from build123d import *

# Parameters (mm, degrees)
F0_R          = 5
F0_R_2        = 4.65
F1_DEPTH      = 0.5
F0_R_3        = 1
F0_R_4        = 0.5
F0_R_5        = 0.15
F2_DEPTH      = 1.7
F2_DEPTH_BACK = 1.2
F3_DEPTH      = 3.4
F3_DEPTH_BACK = 2.9
F5_DEPTH      = 0.3
F6_R          = 0.2414213562
F7_SIZE       = 0.05
F8_SIZE       = 0.15
F9_R          = 0.15
F10_DEPTH     = 1


with BuildPart() as f1:
    # F0 (on Top) → F1 (new body)
    with BuildSketch(Plane.XY):
        Circle(F0_R)
        Circle(F0_R_2, mode=Mode.SUBTRACT)
    extrude(amount=F1_DEPTH)



with BuildPart() as f1b:
    # F0 (on Top) → F1, piece 2 (new body)
    with BuildSketch(Plane.XY):
        Circle(F0_R_3)
        Circle(F0_R_4, mode=Mode.SUBTRACT)
    extrude(amount=F1_DEPTH)

    # F0 (on Top) → F2 (join, two sides)
    with BuildSketch(Plane.XY) as f2_sk:
        Circle(F0_R_4)
        Circle(F0_R_5, mode=Mode.SUBTRACT)
    extrude(amount=F2_DEPTH)
    extrude(f2_sk.sketch, amount=-F2_DEPTH_BACK)

    # F0 (on Top) → F3 (join, two sides)
    with BuildSketch(Plane.XY) as f3_sk:
        Circle(F0_R_5)
    extrude(amount=F3_DEPTH)
    extrude(f3_sk.sketch, amount=-F3_DEPTH_BACK)


with BuildPart() as f1_1:
    add(f1.part)

    add(f1b.part)  # F5 merges F1b
    # F4 (on face) → F5 (join)
    with BuildSketch(Plane.XY):
        with BuildLine():
            Line((-0.3600120544, -0.9329476516), (-0.3600120544, -4.6360426358))
            ThreePointArc((-0.3600120544, -4.6360426358), (0, -4.65), (0.3600120544, -4.6360426358))
            Line((0.3600120544, -4.6360426358), (0.3600120544, -0.9329476516))
            ThreePointArc((0.3600120544, -0.9329476516), (0, -1), (-0.3600120544, -0.9329476516))
        make_face()
        with BuildLine():
            ThreePointArc((0.3600120544, 4.6360426358), (0, 4.65), (-0.3600120544, 4.6360426358))
            Line((-0.3600120544, 4.6360426358), (-0.3600120544, 0.9329476516))
            ThreePointArc((-0.3600120544, 0.9329476516), (0, 1), (0.3600120544, 0.9329476516))
            Line((0.3600120544, 0.9329476516), (0.3600120544, 4.6360426358))
        make_face()
    extrude(amount=F5_DEPTH)

    # F6
    f6_edges = [f1_1.edges().sort_by_distance(p)[0] for p in [
        (-0.5, 0, 0.5),
        (-0.5, 0, 0),
        (-0.15, 0, -1.2),
        (-0.15, 0, 1.7),
    ]]
    fillet(f6_edges, radius=F6_R)

    # F7
    f7_edges = [f1_1.edges().sort_by_distance(p)[0] for p in [
        (-5, 0, 0.5),
        (-4.65, 0, 0.5),
        (-4.65, 0, 0),
        (-5, 0, 0),
    ]]
    chamfer(f7_edges, length=F7_SIZE)

    # F8
    f8_edges = [f1_1.edges().sort_by_distance(p)[0] for p in [
        (-0.15, 0, 3.4),
        (-0.15, 0, -2.9),
    ]]
    chamfer(f8_edges, length=F8_SIZE)

    # F9 (on face) → F10 (join)
    with BuildSketch(Plane.XY):
        with Locations((0, -1.5)):
            Circle(F9_R)
    extrude(amount=-F10_DEPTH)


solid = f1_1.part
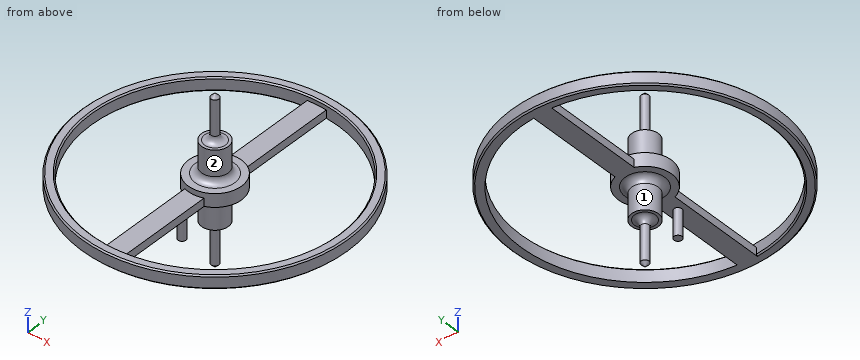
CAD build for the part. Positions are in the model's coordinates, mm. Face numbers are marked on the shaded views. A direction names the side the tool comes from. Give positions to 0.01 mm unless a question says otherwise; leave off trailing zeros. Write each loop counter-clockwise with the first axis right and the second up, starting at its lowest first coordinate (ties: lowest second). Pieces come first, ordered by that corner, then holes. Notation, with made-up numbers: (4, -1.75) -> (31, -1.75) arc R21 cw to (31, 34.25) -> close; hole circle Ø10 at (-0.75, 78.5). An arc over 180 degrees is marked (long way). Return JSON: item names as keys, results as strings.
Item 1: Band-saw the part on B-B (z = 2.5). List the corners of the cut face in (x, y).
Answer below:
{"outline": "circle Ø0.3 at (0, 0)"}
Item 2: Drop flat-ended pins along their axis: pin 1 (3 mm diameter, centred on x = 0, z = 1.5, fed in from -Y); pin 2 (1.5 mm diameter, centred on x = -2, z = 0, fed in from +Y); pin 3 (3 mm diameter, centred on x = -1, y = -3.5, fed in from -Z); pin 4 (5 mm diameter, centred on x = -2, y = 3.5, fed in from +Z). Give the stop position or say it passes through.
Answer below:
{"pin 1": "stops at y = -5", "pin 2": "stops at y = 4.84", "pin 3": "stops at z = 0", "pin 4": "stops at z = 0.5"}
Item 3: Band-saw the part on D-D (z = 1.5). List the corners of the cut face in (x, y), then the cut area to 3 significant figures.
Answer below:
{"outline": "circle Ø1 at (0, 0)", "area": "0.785 mm2"}
Item 4: Band-saw the part on A-A (y = -4.5). Give the number of separate pieces and of enclosed holes in the cut face, then the cut area to 3 significant figures.
Answer below:
{"separate pieces": "3", "enclosed holes": "0", "area": "1.20 mm2"}
Item 5: Tool access for the marked faces 1 and 2: list every direction of +Z, -Z, +X, -X, +Y, -Y with a clear straight run to the whole face (end or side of a thin tool).
Answer below:
{"face 1": "-Z", "face 2": "+Z"}
Item 6: Drill centre lines: probe 1 along Y at (x, z) = (-0.5, 0.25); probe 2 along Z at (x, y) = (0.5, -0.75). Where is each one in solid material? Low to high.
Answer below:
{"probe 1": "y = -4.97 to -4.62, -0.87 to 0.87, 4.62 to 4.97", "probe 2": "z = 0 to 0.5"}
